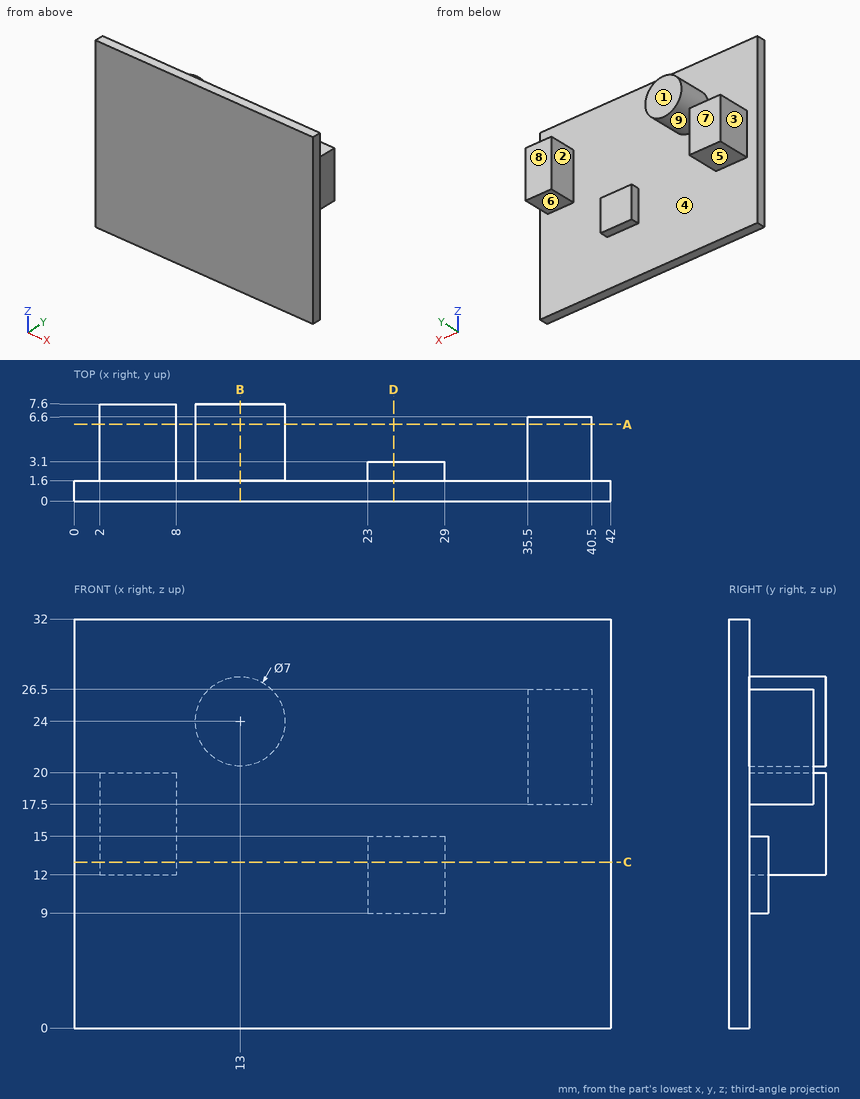
For this review, use the dimensioned drawing (mm, ordinates from the lowest corner) and the shaded views. A direction names the side the tool comes from. Coordinates: 2 decimals unless noted, no trailing zeros. Order: outer loops, then holes, each group sorted by start corner. A loop starts at its lowest first (then second) coordinate and runs counter-clockwise, first axis right, second up. Notation, with made-up numbers: (38, 38.25) - (93, 38.25) arc R31 ccw to (93, 70.25) - close; hole circle Ø6 at (-18, 43.25). An arc over 180 degrees is marked (long way). Answer as a JSON object with one key per item and string values. Group by question number.
1. We need section B-B on x = 13. State the section outline as (y, z) points.
2. We need section A-A on y = 6. State the section outline as (x, z) points.
3. Clearance check with flat-ended pins moving along their axes: P1, Ø3, axis at x = 29.5, z = 7, coming from the +Y side; P2, Ø0.8, axis at y = 2.5, z = 12, coming from the -X side; P3, Ø5.5, axis at x = 37, z = 24, coming from the +Y side. State where each tip first meets the part, or that it passes through.
4. We need section D-D on x = 25. State the section outline as (y, z) points, then the cut area to 3 significant figures.
5. For probe 1 along Y at (x, z) = (9.5, 16.5); probe 2 along Z at (x, y) = (13, 7); probe 3 along Z at (x, y) = (36, 4.75), list the stretches that pass through material, from the lowest coordinate up.
6. The part is to be moulded in two halves that separate along X. For the marked faces 1, 2, 3 and 4, say which applies: pulls with the +X half, pulls with the -X half, needs draft (parallel to the pull), parting line crosses it, or undercut.
7. We need section C-C on z = 13. State the section outline as (x, y) points.
8. For the marked faces 5, 6, 7, 8 and 9, list the 3-axis set-ups (+Z, -Z, +X, -X, +Y, -Y) from which the entire face can be reached by the end or side of a thin tool; tool diameter is ignored.
Final values:
{
 "1": {"outline": "(0, 0) - (1.6, 0) - (1.6, 20.5) - (7.6, 20.5) - (7.6, 27.5) - (1.6, 27.5) - (1.6, 32) - (0, 32) - close"},
 "2": {"outline": "(2, 12) - (8, 12) - (8, 20) - (2, 20) - close; circle Ø7 at (13, 24); (35.5, 17.5) - (40.5, 17.5) - (40.5, 26.5) - (35.5, 26.5) - close"},
 "3": {"P1": "y = 1.6", "P2": "x = 2", "P3": "y = 6.6"},
 "4": {"outline": "(0, 0) - (1.6, 0) - (1.6, 9) - (3.1, 9) - (3.1, 15) - (1.6, 15) - (1.6, 32) - (0, 32) - close", "area": "60.2 mm²"},
 "5": {"probe 1": "0 to 1.6", "probe 2": "20.5 to 27.5", "probe 3": "17.5 to 26.5"},
 "6": {"face 1": "needs draft", "face 2": "undercut", "face 3": "pulls with the -X half", "face 4": "undercut"},
 "7": {"outline": "(0, 0) - (42, 0) - (42, 1.6) - (29, 1.6) - (29, 3.1) - (23, 3.1) - (23, 1.6) - (8, 1.6) - (8, 7.6) - (2, 7.6) - (2, 1.6) - (0, 1.6) - close"},
 "8": {"face 5": "-Z, -X, +Y", "face 6": "-Z, +X, +Y", "face 7": "+Z, -Z, +X, -X, +Y", "face 8": "+Z, -Z, +X, +Y", "face 9": "+Y"}
}
